Autodesk Inventor part; units mm, degrees
ref_plane "YZ Plane" through (0, 0, 0) normal (1, 0, 0) x (0, 1, 0)
ref_plane "XZ Plane" through (0, 0, 0) normal (0, 1, 0) x (-1, 0, 0)
ref_plane "XY Plane" through (0, 0, 0) normal (0, 0, 1) x (1, 0, 0)
sketch "Skizze2" plane through (0, 0, 0) normal (0, 1, 0) x (-1, 0, 0)
  line L0 (15.4, 0) -> (-15.4, 0)
  line L1 (0, -0.6) -> (0, 3.6)
  line L2 (-11, 0) -> (11, 0)
  line L3 (11, 0) -> (11, 2.5)
  line L4 (-11, 2.5) -> (-11, 0)
  line L5 (-9, 3) -> (-9, 2.85)
  line L6 (-9, 2.85) -> (-9.8, 2.85)
  line L7 (-9.8, 2.85) -> (-9.8, 3)
  line L8 (9, 3) -> (9, 2.85)
  line L9 (9, 2.85) -> (9.8, 2.85)
  line L10 (9.8, 2.85) -> (9.8, 3)
  line L11 (-9.8, 3) -> (-10.5, 3)
  line L12 (10.5, 3) -> (9.8, 3)
  line L13 (9, 3) -> (-9, 3)
  line L14 (-11, 2.5) -> (-10.5, 3)
  line L15 (11, 2.5) -> (10.5, 3)
  point P0 (0, 0)
  point P1 (11, 3)
  point P2 (-11, 3)
  dimension "d3" = 6
  dimension "d4" = 5.7
  dimension "d5" = 22
  dimension "d6" = 18
  dimension "d7" = 0.8
  dimension "d8" = 0.5
  dimension "d9" = 0.5
  dimension "d10" = 0.5
  dimension "d11" = 0.5
revolve "Umdrehung1" add sketch "Skizze2" angle 360 about axis through (-10, 0, 0) along (1, 0, 0)
properties part number "13_0204_054"
The listing builds one solid part. Answer for the finished solid, in the listing's coordinates (mm). Give positions to 0.01 mm unless a question says otherwise; leave off trailing zeros. Order: outer loops, then holes, each group sorted by start corner. A loop starts at its lowest first (then second) coordinate and runs counter-clockwise, first axis right, second up. Notation, with made-up numbers: (20, 1) - (65, 1) arc R24 cw to (65, 18) - close; hole circle Ø1 at (-5, 13). An arc over 180 degrees is marked (long way). One line per item, written item: value. Start each with the question number.
1) A cutting plane is placed at B-B on x = -2.25. Give the vertices of the cut face in (y, z).
2) The mould has two halves that part along X. Classify faces 1 (the face through (-10, 0, -3)), 2 (the face through (9.406, 1.734, -2.262)), 3 (the face through (-11, 0, 0)), 4 (the face through (-9.406, -1.734, -2.262)): released by +X, released by -X, zero draft, split by the parting line, or undercut.
3) Find the intervals of material crossed by L1, parallel to Z at x = -8.25, y = 1.65; L2, parallel to Z at x = 9.25, y = 2.55; L3, parallel to Y at x = 10, z = 1.1, in increasing order.
4) A cutting plane is placed at A-A on x = 9.5. Give the vertices of the cut face in (y, z), then the cut area to 3 significant figures.
Answer sheet:
1. outline: circle Ø6 at (0, 0)
2. face 1: zero draft
2. face 2: undercut
2. face 3: released by -X
2. face 4: undercut
3. L1: z = -2.51 to 2.51
3. L2: z = -1.27 to 1.27
3. L3: y = -2.79 to 2.79
4. outline: circle Ø5.7 at (0, 0)
4. area: 25.5 mm2
